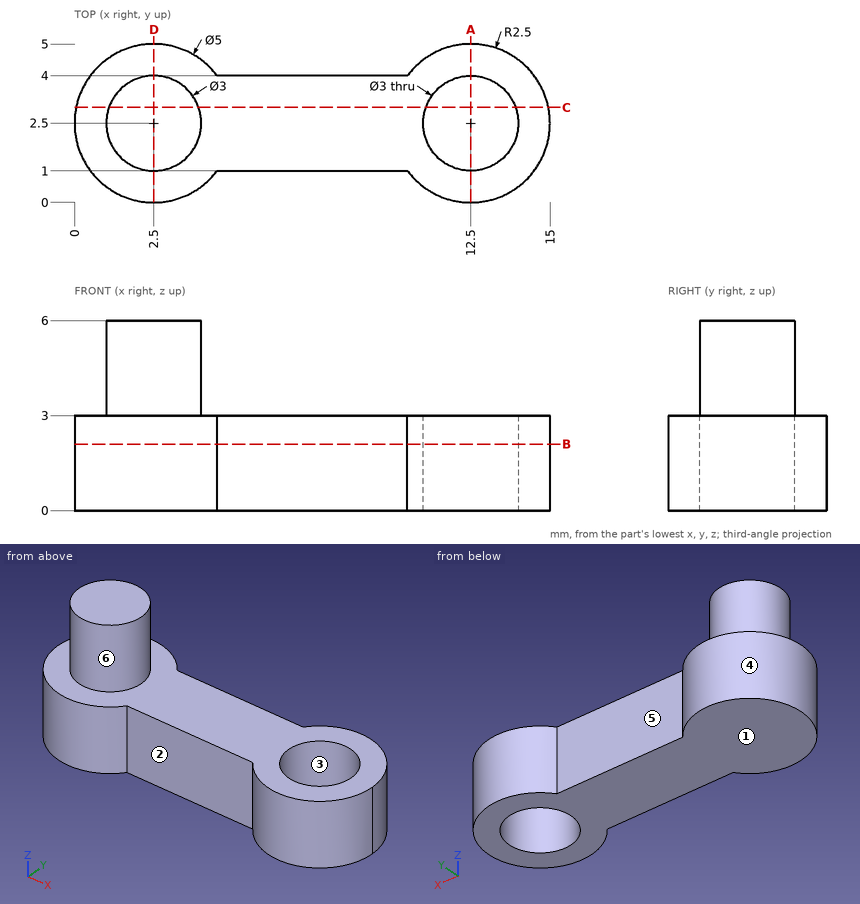
Geometry check sheet. Reference: drawing and pictorial views, mm from the part's lowest x, y, z. A direction names the side the tool comes from. Round coordinates to 2 decimals unless told otherwise and drop trailing zeros. Loops run counter-clockwise (first coordinate to the right, second up) from the corner with the lowest first, then second, coordinate; pieces in that order, holes last. Notation, with made-up numbers: M 46,29 L 52,29 A27 cw 52,48 Z; hole C 30.25,45.5 d1. An arc over 180 degrees is marked long. Return JSON: item names as keys, results as strings. Group by question number.
(1) Set-up check for the marked faces 4, 5 and 6: record each of +Z, -Z, +X, -X, +Y, -Y from which the full face is reachable in a straight line by a thin tool's end or side.
(2) Go/stop test with flat-tipped pins: pin 1 (2.5 mm diameter, centred on x = 6.5, z = 2, fed in from +Y); pin 2 (1.5 mm diameter, centred on x = 8.5, z = 2, fed in from -Y); pin 3 (1 mm diameter, centred on x = 4, z = 4.5, fed in from -Y); pin 4 (2.5 mm diameter, centred on x = 12.5, y = 2.5, fed in from -Z). Record where each tip stops, or that it passes through.
(3) Section check D-D, the plane x = 2.5. Enter the section's corners in (y, z).
(4) Scan lines: line 1 along Y through (x, z) = (12.5, 0.8); line 2 along Z through (x, y) = (10.25, 2.4); line 3 along X through (y, z) = (0.2, 0.4). Record each from-to range of solid material in increasing order. Write a range as [from, to].
(5) Section check A-A, the plane x = 12.5. Enter the section's corners in (y, z), and give its area (3 significant figures).
(6) Mould release check, pull along Y, two halves, no side actions. Record for the marked faces 1, 2 and 3: pulls with the +Y half, pulls with the -Y half, needs draft (parallel to the pull), parting line crosses it, or undercut.
(7) Section check B-B, the plane z = 2.1. Enter the section's corners in (x, y).
(8) Section check C-C, the plane y = 3. Enter the section's corners in (x, z).
Data:
{
 "1": {"face 4": "+Z, -Z", "face 5": "+Z, -Z, +Y", "face 6": "+Z"},
 "2": {"pin 1": "y = 4", "pin 2": "y = 1", "pin 3": "y = 1.38", "pin 4": "through"},
 "3": {"outline": "M 0,0 L 5,0 L 5,3 L 4,3 L 4,6 L 1,6 L 1,3 L 0,3 Z"},
 "4": {"line 1": "[0, 1], [4, 5]", "line 2": "[0, 3]", "line 3": "[1.52, 3.48], [11.52, 13.48]"},
 "5": {"outline": "M 0,0 L 1,0 L 1,3 L 0,3 Z; M 4,0 L 5,0 L 5,3 L 4,3 Z", "area": "6.00 mm²"},
 "6": {"face 1": "needs draft", "face 2": "pulls with the -Y half", "face 3": "undercut"},
 "7": {"outline": "M 4.5,1 L 10.5,1 A2.5 ccw long 10.5,4 L 4.5,4 A2.5 ccw long Z; hole C 12.5,2.5 d3"},
 "8": {"outline": "M 0.05,0 L 11.09,0 L 11.09,3 L 3.91,3 L 3.91,6 L 1.09,6 L 1.09,3 L 0.05,3 Z; M 13.91,0 L 14.95,0 L 14.95,3 L 13.91,3 Z"}
}
